The model under review builds one solid part; all positions refer to its coordinate system, in mm. A direction names the side the tool comes from. Coordinates: 2 decimals unless noted, no trailing zeros. Write each loop counter-clockwise with the first axis right and the second up, starting at its lowest first coordinate (ties: lowest second). Pieces come first, ordered by that corner, then holes. Notation, with made-up numbers: M 78.5,-29.75 L 94.5,-29.75 A28 ccw 94.5,4.25 Z; hole C 0,-19 d10. An arc over 180 degrees is marked long. Answer as a JSON object with one key per item and string values.
```python
from build123d import *

# Parameters (mm, degrees)
BOSS_EXTRUDE1_DEPTH = 3
CUT_EXTRUDE1_DEPTH  = 1
SKETCH3_R           = 0.8
CUT_EXTRUDE2_DEPTH  = 4


with BuildPart() as part:
    # Sketch1 → Boss-Extrude1 (new body)
    with BuildSketch(Plane(origin=(0, 0, 0), x_dir=(1, 0, 0), z_dir=(0, 1, 0))):
        with BuildLine():
            Line((21.25, -8.375), (21.25, 8.375))
            ThreePointArc((21.25, 8.375), (20.407931996, 10.407931996), (18.375, 11.25))
            Line((18.375, 11.25), (-15.25, 11.25))
            ThreePointArc((-15.25, 11.25), (-17.282931996, 10.407931996), (-18.125, 8.375))
            Line((-18.125, 8.375), (-18.125, -8.375))
            ThreePointArc((-18.125, -8.375), (-17.282931996, -10.407931996), (-15.25, -11.25))
            Line((-15.25, -11.25), (18.375, -11.25))
            ThreePointArc((18.375, -11.25), (20.407931996, -10.407931996), (21.25, -8.375))
        make_face()
    extrude(amount=BOSS_EXTRUDE1_DEPTH)

    # Sketch2 → Cut-Extrude1 (cut)
    with BuildSketch(Plane(origin=(0, 3, 0), x_dir=(1, 0, 0), z_dir=(0, 1, 0))):
        with BuildLine():
            ThreePointArc((18.375, -11.25), (20.407931996, -10.407931996), (21.25, -8.375))
            Line((21.25, -8.375), (21.25, 8.375))
            ThreePointArc((21.25, 8.375), (20.407931996, 10.407931996), (18.375, 11.25))
            Line((18.375, 11.25), (-15.25, 11.25))
            ThreePointArc((-15.25, 11.25), (-17.282931996, 10.407931996), (-18.125, 8.375))
            Line((-18.125, 8.375), (-18.125, -8.375))
            ThreePointArc((-18.125, -8.375), (-17.282931996, -10.407931996), (-15.25, -11.25))
            Line((-15.25, -11.25), (18.375, -11.25))
        make_face()
        with BuildLine():
            Line((-13.75, -4.15), (-13.75, 4.15))
            ThreePointArc((-13.75, 4.15), (-13.354594155, 5.104594155), (-12.4, 5.5))
            Line((-12.4, 5.5), (12.4, 5.5))
            ThreePointArc((12.4, 5.5), (13.354594155, 5.104594155), (13.75, 4.15))
            Line((13.75, 4.15), (13.75, -4.15))
            ThreePointArc((13.75, -4.15), (13.354594155, -5.104594155), (12.4, -5.5))
            Line((12.4, -5.5), (-12.4, -5.5))
            ThreePointArc((-12.4, -5.5), (-13.354594155, -5.104594155), (-13.75, -4.15))
        make_face(mode=Mode.SUBTRACT)
    extrude(amount=-CUT_EXTRUDE1_DEPTH, mode=Mode.SUBTRACT)

    # Sketch3 → Cut-Extrude2 (cut, through all)
    with BuildSketch(Plane.XZ):
        with Locations((-12.935284159, -7.779032038)):
            Circle(SKETCH3_R)
        with Locations((-12.935284159, 8.720967962)):
            Circle(SKETCH3_R)
        with Locations((17.064715841, -7.779032038)):
            Circle(SKETCH3_R)
        with Locations((17.064715841, 8.720967962)):
            Circle(SKETCH3_R)
    extrude(amount=-CUT_EXTRUDE2_DEPTH, mode=Mode.SUBTRACT)


solid = part.part
```
(1) For faces 5 (the face through (20.385, 0.986, 10.43)), 6 (the face through (-13.75, 2.5, 0.1)), 7 (the face through (21.25, 1, 0)), 8 (the face through (-13.34, 2.51, 5.12)), 9 (the face through (0.2, 2.5, 5.5)), list the 3-axis set-ups (+Z, -Z, +X, -X, +Y, -Y) from which the entire face can be reached by the end or side of a thin tool; tool diameter is ignored.
Results list:
{"face 5": "+Z, +X, +Y, -Y", "face 6": "+Z, -Z, -X, +Y", "face 7": "+Z, -Z, +X, +Y, -Y", "face 8": "+Z, -X, +Y", "face 9": "+Z, +X, -X, +Y"}
(2) Draft analysis for pull direction X (two halves, no side actions). For faces 1 (the face through (1, 2, -8)), 2 (the face through (-12.17, 0.99, 8.96)), 3 (the face through (13.37, 2.51, 5.09)), 4 (the face through (-17.305, 0.986, 10.385)), state which applies: released by +X, released by -X, zero draft, split by the parting line, or undercut.
Results list:
{"face 1": "zero draft", "face 2": "undercut", "face 3": "released by +X", "face 4": "released by -X"}
(3) For pin 1 Ø6 at (x, z) = (-6.5, -9) entering from +Y, flat-tipped, find the tip position at first contact; note if it passes through.
Results list:
{"pin 1": "y = 2"}
(4) Add section B-B on x = -0.5. Give the boundary of the cut face in (y, z).
Results list:
{"outline": "M 0,-11.25 L 2,-11.25 L 2,-5.5 L 3,-5.5 L 3,5.5 L 2,5.5 L 2,11.25 L 0,11.25 Z"}
(5) Add section D-D on z = 7.25. Give the boundary of the cut face in (x, y) (3 decimals), and give its area (4 significant figures).
Results list:
{"outline": "M -18.125,0 L 21.25,0 L 21.25,2 L -18.125,2 Z", "area": "78.75 mm²"}
(6) Wall thickness on line 1 along X through (y, z) = (0.3, 9.25); line 2 along Z through (x, y) = (11.5, 2.3); line 3 along Y through (x, z) = (8, -8): over which ranges is each line inside the solid? List them lowest first. Write a range as from..to.
Results list:
{"line 1": "-17.99..-13.54, -12.34..16.46, 17.66..21.11", "line 2": "-5.5..5.5", "line 3": "0..2"}
(7) Add section A-A on z = 1.5. Give the boundary of the cut face in (x, y) (3 decimals), and give its area (3 significant figures).
Results list:
{"outline": "M -18.125,0 L 21.25,0 L 21.25,2 L 13.75,2 L 13.75,3 L -13.75,3 L -13.75,2 L -18.125,2 Z", "area": "106 mm²"}
(8) Add section C-C on y = 1.1. Give the boundary of the cut face in (x, z) (3 decimals), and give its area (3 significant figures).
Results list:
{"outline": "M -18.125,-8.375 A2.875 ccw -15.25,-11.25 L 18.375,-11.25 A2.875 ccw 21.25,-8.375 L 21.25,8.375 A2.875 ccw 18.375,11.25 L -15.25,11.25 A2.875 ccw -18.125,8.375 Z; hole C -12.935,-7.779 d1.6; hole C -12.935,8.721 d1.6; hole C 17.065,-7.779 d1.6; hole C 17.065,8.721 d1.6", "area": "871 mm²"}
